Model file for the job. Use its own axes, mm. Face numbers are marked on the shaded views. A direction names the side the tool comes from. Round coordinates to 2 decimals unless told otherwise and drop trailing zeros. Loops run counter-clockwise (first coordinate to the right, second up) from the corner with the lowest first, then second, coordinate; pieces in that order, holes last. Notation, with made-up numbers: M 33.25,-32.5 L 47.25,-32.5 A36 ccw 47.25,3.5 Z; hole C 76.25,-20.5 d8. An arc over 180 degrees is marked long. Use a Markdown table: item, result. Add a question column.
Q1. Cut at D-D (y = -6). Give the cut face in (x, z).
Q2. Pin check, flat tip, straight feed: pin 1 (20 mm diameter, centred on y = -43.5, z = 15.5, fed in from -X). Stop position of the tip, or through.
Q3. Cut at C-C (z = 29). Give the cut face in (x, y).
Q4. Tool access for the marked faces 1, 2, 3, 4 and 5: list every direction of +Z, -Z, +X, -X, +Y, -Y with a clear straight run to the whole face (end or side of a thin tool).
Q5. Cut at A-A (z = 20.5). State how many separate pieces and enclosed holes the cut face has, plus the area to 3 significant figures.
Q6. Probe line 1 (Y direction, x = 3.5, z = 69.31); line 2 (Y direction, x = 3.5, z = 7.5); line 3 (Z direction, x = -1.75, y = -50.5). List the from-to ranges inside material, lowest first. Write a range as from..to.
Q7. Mould opens along Y. For the marked faces 6, 7 and 8 say: +Y half, -Y half, draft (parallel to the pull), parting line (faces both ways), or undercut.
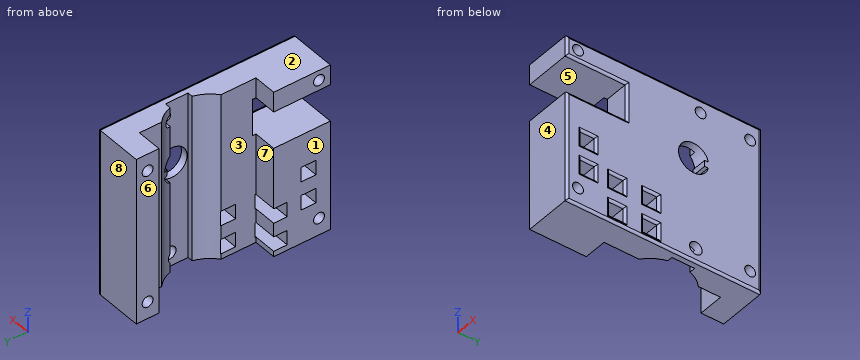
from build123d import *

# Parameters (mm, degrees)
PROFILEEXTRUDE_DEPTH = 73.76
HOSEWINDOW_W         = 16.29
HOSEWINDOW_H         = 26.5
HOSEWINDOWCUT_DEPTH  = 22.63
CAGESCREWS_R         = 2.4
CAGESCREWSCUT_DEPTH  = 22.63
AXLEHOLECUT_DEPTH    = 22.63
SETSCREWS_R          = 2.426338021
SETSCREWS_R_2        = 2.788762315
SETSCREWSCUT_DEPTH   = 22.63
SKETCH1_W            = 6.5
SKETCH1_H            = 6.5
CUT_EXTRUDE1_DEPTH   = 22.63
FILLET1_R            = 1


with BuildPart() as part:
    # Profile → ProfileExtrude (new body)
    with BuildSketch(Plane.XY):
        with BuildLine():
            Line((-6.01073477, -58.62791746), (-6.01073477, -33.62791746))
            Line((-6.01073477, -33.62791746), (4.13926523, -33.62791746))
            Line((4.13926523, -33.62791746), (4.13926523, -18.13791746))
            ThreePointArc((4.13926523, -18.13791746), (7.563334043, -14.326029686), (9.63126523, -9.63791746))
            Line((9.63126523, -9.63791746), (11.94926523, -9.63791746))
            Line((11.94926523, -9.63791746), (11.94926523, 0.36208254))
            Line((11.94926523, 0.36208254), (9.35926523, 0.36208254))
            ThreePointArc((9.35926523, 0.36208254), (7.525939238, 4.313848402), (4.70926523, 7.63708254))
            Line((4.70926523, 7.63708254), (4.70926523, 17.41208254))
            Line((4.70926523, 17.41208254), (-6.44073477, 17.41208254))
            Line((-6.44073477, 17.41208254), (-6.44073477, 27.41208254))
            Line((-6.44073477, 27.41208254), (15.18926523, 27.41208254))
            Line((15.18926523, 27.41208254), (15.18926523, -58.62791746))
            Line((15.18926523, -58.62791746), (-6.01073477, -58.62791746))
        make_face()
    extrude(amount=PROFILEEXTRUDE_DEPTH)

    # HoseWindow → HoseWindowCut (cut, through all)
    with BuildSketch(Plane(origin=(15.18926523, 0, 0), x_dir=(0, 0, -1), z_dir=(1, 0, 0))):
        with Locations((-56.725, -45.37791746)):
            Rectangle(HOSEWINDOW_W, HOSEWINDOW_H)
    extrude(amount=-HOSEWINDOWCUT_DEPTH, mode=Mode.SUBTRACT)

    # CageScrews → CageScrewsCut (cut, through all)
    with BuildSketch(Plane(origin=(15.18926523, 0, 0), x_dir=(0, 0, -1), z_dir=(1, 0, 0))):
        with Locations((-66.26, 22.41208254)):
            Circle(CAGESCREWS_R)
        with Locations((-7.5, 22.41208254)):
            Circle(CAGESCREWS_R)
        with Locations((-7.5, -53.62791746)):
            Circle(CAGESCREWS_R)
        with Locations((-69.31, -53.62791746)):
            Circle(CAGESCREWS_R)
    extrude(amount=-CAGESCREWSCUT_DEPTH, mode=Mode.SUBTRACT)

    # AxleHole → AxleHoleCut (cut, through all)
    with BuildSketch(Plane(origin=(15.18926523, 0, 0), x_dir=(0, 0, -1), z_dir=(1, 0, 0))):
        with BuildLine():
            Line((-44.699, 2.307293484), (-47.361, 2.307293484))
            Line((-47.361, 2.307293484), (-47.361, 3.926293484))
            ThreePointArc((-47.361, 3.926293484), (-46.03, -9.21691746), (-44.699, 3.926293484))
            Line((-44.699, 3.926293484), (-44.699, 2.307293484))
        make_face()
    extrude(amount=-AXLEHOLECUT_DEPTH, mode=Mode.SUBTRACT)

    # SetScrews → SetScrewsCut (cut, through all)
    with BuildSketch(Plane(origin=(15.18926523, 0, 0), x_dir=(0, 0, -1), z_dir=(1, 0, 0))):
        with Locations((-67.80722939, 0.544946624)):
            Circle(SETSCREWS_R)
        with Locations((-6.04299884, -1.55824191)):
            Circle(SETSCREWS_R_2)
    extrude(amount=-SETSCREWSCUT_DEPTH, mode=Mode.SUBTRACT)

    # Sketch1 → Cut-Extrude1 (cut, through all)
    with BuildSketch(Plane(origin=(15.18926523, 0, 0), x_dir=(0, 0, -1), z_dir=(1, 0, 0))):
        with Locations((-18.25, -49.02791746)):
            Rectangle(SKETCH1_W, SKETCH1_H)
        with Locations((-30.85, -49.02791746)):
            Rectangle(SKETCH1_W, SKETCH1_H)
        with Locations((-5.65, -36.32791746)):
            Rectangle(SKETCH1_W, SKETCH1_H)
        with Locations((-18.25, -36.32791746)):
            Rectangle(SKETCH1_W, SKETCH1_H)
        with Locations((-5.65, -21.32791746)):
            Rectangle(SKETCH1_W, SKETCH1_H)
        with Locations((-18.25, -21.32791746)):
            Rectangle(SKETCH1_W, SKETCH1_H)
    extrude(amount=-CUT_EXTRUDE1_DEPTH, mode=Mode.SUBTRACT)

    # Fillet1
    fillet1_edges = [part.edges().sort_by_distance(p)[0] for p in [
        (15.18926523, -45.77791746, 18.25),
        (15.18926523, -49.02791746, 21.5),
        (15.18926523, -52.27791746, 18.25),
        (15.18926523, -49.02791746, 15),
        (15.18926523, -49.02791746, 34.1),
        (15.18926523, -52.27791746, 30.85),
        (15.18926523, -49.02791746, 27.6),
        (15.18926523, -45.77791746, 30.85),
        (15.18926523, -36.32791746, 8.9),
        (15.18926523, -39.57791746, 5.65),
        (15.18926523, -36.32791746, 2.4),
        (15.18926523, -33.07791746, 5.65),
        (15.18926523, -15.60791746, 0),
        (15.18926523, -36.32791746, 21.5),
        (15.18926523, -39.57791746, 18.25),
        (15.18926523, -36.32791746, 15),
        (15.18926523, -33.07791746, 18.25),
        (15.18926523, -21.32791746, 8.9),
        (15.18926523, -24.57791746, 5.65),
        (15.18926523, -21.32791746, 2.4),
        (15.18926523, -18.07791746, 5.65),
        (15.18926523, -58.62791746, 69.315),
        (15.18926523, -21.32791746, 21.5),
        (15.18926523, -24.57791746, 18.25),
        (15.18926523, -21.32791746, 15),
        (15.18926523, -18.07791746, 18.25),
        (15.18926523, 27.41208254, 36.88),
        (15.18926523, -58.62791746, 24.29),
        (15.18926523, -15.60791746, 73.76),
        (15.18926523, -45.37791746, 64.87),
        (15.18926523, -45.37791746, 48.58),
        (15.18926523, -32.12791746, 56.725),
    ]]
    fillet(fillet1_edges, radius=FILLET1_R)


solid = part.part
Checked values:
| question | item | result |
|---|---|---|
| 1 | outline | M 11.95,0 L 14.19,0 A1 ccw 15.19,1 L 15.19,40.34 L 11.95,40.34 Z; M 11.95,51.72 L 15.19,51.72 L 15.19,72.76 A1 ccw 14.19,73.76 L 11.95,73.76 Z |
| 2 | pin 1 | stops at x = -6.01 |
| 3 | outline | M -6.44,17.41 L 4.71,17.41 L 4.71,7.64 A16.26 cw 9.36,0.36 L 11.95,0.36 L 11.95,-9.64 L 9.63,-9.64 A16.26 cw 4.14,-18.14 L 4.14,-33.63 L -6.01,-33.63 L -6.01,-45.78 L 14.19,-45.78 A1 ccw 15.19,-44.78 L 15.19,26.41 A1 ccw 14.19,27.41 L -6.44,27.41 Z; M -6.01,-58.63 L 14.19,-58.63 A1 ccw 15.19,-57.63 L 15.19,-53.28 A1 ccw 14.19,-52.28 L -6.01,-52.28 Z |
| 4 | face 1 | +Z, -Z, -X, -Y |
| 4 | face 2 | +Z, +X, -X, +Y, -Y |
| 4 | face 3 | +Z, -Z, -X |
| 4 | face 4 | +Z, -Z, +X, -X, -Y |
| 4 | face 5 | +X, -X, -Y |
| 5 | separate pieces | 4 |
| 5 | enclosed holes | 0 |
| 5 | area | 830 mm^2 |
| 6 | line 1 | y = -58.63..-56.03, -51.23..-33.63, 17.41..27.41 |
| 6 | line 2 | y = -58.63..-56.03, -51.23..-39.58, 17.41..20.01, 24.81..27.41 |
| 6 | line 3 | z = 0..15, 21.5..27.6, 34.1..48.58, 64.87..73.76 |
| 7 | face 6 | draft |
| 7 | face 7 | undercut |
| 7 | face 8 | +Y half |
